from build123d import *

# Parameters (mm, degrees)
SKETCH_1_R          = 2.5
SKETCH_1_R_2        = 3
EXTRUDE_1_DEPTH     = 5
SKETCH_2_R          = 10
SKETCH_2_R_2        = 3
EXTRUDE_2_DEPTH     = 5
FILLET_1_R          = 0.3
CHAMFER_1_SIZE      = 0.5
CUT_EXTRUDE_1_REACH = 29.325
SKETCH_3_W          = 1
SKETCH_3_H          = 13.579366256
HOLE_WIZARD_M4_1_D  = 3.3


with BuildPart() as part:
    # 草图1 → 凸台-拉伸1 (new body)
    with BuildSketch(Plane(origin=(0, 0, 0), x_dir=(1, 0, 0), z_dir=(0, 1, 0))):
        with BuildLine():
            Line((-17.966197006, 5.136542547), (-7.985903938, 8.956859846))
            Line((-7.985903938, 8.956859846), (-7.985903938, 13.579366256))
            Line((-7.985903938, 13.579366256), (7.985903938, 13.579366256))
            Line((7.985903938, 13.579366256), (7.985903938, 8.956859846))
            Line((7.985903938, 8.956859846), (17.966197006, 5.136542547))
            ThreePointArc((17.966197006, 5.136542547), (21.495547327, -0.221268111), (17.546875, -5.277989933))
            Line((17.546875, -5.277989933), (1.435216594, -10))
            Line((1.435216594, -10), (-1.435216594, -10))
            Line((-1.435216594, -10), (-17.546875, -5.277989933))
            ThreePointArc((-17.546875, -5.277989933), (-21.495547327, -0.221268111), (-17.966197006, 5.136542547))
        make_face()
        with Locations(Location((-16, 0, 0), (0, 0, 270))):
            Circle(SKETCH_1_R, mode=Mode.SUBTRACT)
        with Locations(Location((0, 0, 0), (0, 0, 270))):
            Circle(SKETCH_1_R_2, mode=Mode.SUBTRACT)
        with Locations(Location((16, 0, 0), (0, 0, 90))):
            Circle(SKETCH_1_R, mode=Mode.SUBTRACT)
    extrude(amount=EXTRUDE_1_DEPTH)

    # 草图2 → 凸台-拉伸2 (add)
    with BuildSketch(Plane(origin=(0, 5, 0), x_dir=(1, 0, 0), z_dir=(0, 1, 0))):
        with Locations(Location((0, 0, 0), (0, 0, 270))):
            Circle(SKETCH_2_R)
        with Locations(Location((0, 0, 0), (0, 0, 270))):
            Circle(SKETCH_2_R_2, mode=Mode.SUBTRACT)
    extrude(amount=EXTRUDE_2_DEPTH)

    # 圆角1
    fillet_1_edges = [part.edges().sort_by_distance(p)[0] for p in [
        (0, 0, -13.579366256),
        (7.985903938, 0, -11.268113051),
        (-7.985903938, 2.5, -13.579366256),
        (7.985903938, 2.5, -13.579366256),
        (7.985903938, 5, -11.268113051),
        (0, 5, -13.579366256),
        (-7.985903938, 5, -11.268113051),
        (-7.985903938, 0, -11.268113051),
    ]]
    fillet(fillet_1_edges, radius=FILLET_1_R)

    # 倒角1
    chamfer_1_edges = [part.edges().sort_by_distance(p)[0] for p in [
        (0, 10, -10),
    ]]
    chamfer(chamfer_1_edges, length=CHAMFER_1_SIZE)

    # 草图3 → 切除-拉伸1 (cut, up to next)
    with BuildSketch(Plane(origin=(0, 10, 0), x_dir=(1, 0, 0), z_dir=(0, 1, 0)), mode=Mode.PRIVATE) as cut_extrude_1_sk1:
        with Locations((0, 6.789683128)):
            Rectangle(SKETCH_3_W, SKETCH_3_H)
    cut_extrude_1_tool1 = extrude(cut_extrude_1_sk1.sketch, amount=-CUT_EXTRUDE_1_REACH, mode=Mode.PRIVATE) & part.part
    add(cut_extrude_1_tool1.solids().sort_by_distance((0, 10, -6.789683))[0], mode=Mode.SUBTRACT)

    # M4 螺纹孔1 (through all)
    with Locations(Plane(origin=(-7.985903938, 2.5, -11.156859846), x_dir=(0, 0, -1), z_dir=(-1, 0, 0))):
        with Locations((0, 0)):
            Hole(HOLE_WIZARD_M4_1_D / 2)


solid = part.part
The listing builds one solid part. Answer for the finished solid, in the listing's coordinates (mm). A direction names the side the tool comes from. Give positions to 0.01 mm unless a question says otherwise; leave off trailing zeros. Write each loop counter-clockwise with the first axis right and the second up, starting at its lowest first coordinate (ties: lowest second). Pieces come first, ordered by that corner, then holes. Notation, with made-up numbers: (48, 10) - (57, 10) arc R20 ccw to (57, 25) - close; hole circle Ø3 at (31.25, 36.25). An arc over 180 degrees is marked (long way). Use a Markdown table: item, result.
1. For a pull along Y with two mould halves and no side action, classify faces 1 (the cylindrical face through (-18.44, 2.46, -0.54)), 2 (the cylindrical face through (4.295, 2.427, -12.805)), 3 (the flat face through (2.24, 10, -2.24)), 4 (the cylindrical face through (-4.191, 2.427, -12.805)) as released by +Y, released by -Y, zero draft, split by the parting line, or undercut.
Values follow:
| item | result |
|---|---|
| face 1 | zero draft |
| face 2 | undercut |
| face 3 | released by +Y |
| face 4 | undercut |
2. Find the intervals of material crossed by probe 1 along X at (y, z) = (2.8, 0); probe 2 along Y at (x, z) = (12.5, -4.5); probe 3 along Z at (x, y) = (-1.5, 1.5), in increasing order. Write a range as from..to.
Values follow:
| item | result |
|---|---|
| probe 1 | x = -21.5..-18.5, -13.5..-3, 3..13.5, 18.5..21.5 |
| probe 2 | y = 0..5 |
| probe 3 | z = -13.58..-12.47, -9.84..-2.6, 2.6..9.98 |
3. Section A-A on y = 2.5 is taken. Write down the section's boundary in (x, z), plus the area to 3 significant figures.
Values follow:
| item | result |
|---|---|
| outline | (-17.97, -5.14) - (-7.99, -8.96) - (-7.99, -9.51) - (-0.5, -9.51) - (-0.5, -2.96) arc R3 cw (long way) to (0.5, -2.96) - (0.5, -9.51) - (7.99, -9.51) - (7.99, -8.96) - (17.97, -5.14) arc R5.5 ccw to (17.55, 5.28) - (1.44, 10) - (-1.44, 10) - (-17.55, 5.28) arc R5.5 ccw to start; (-7.99, -13.28) arc R0.3 ccw to (-7.69, -13.58) - (-0.5, -13.58) - (-0.5, -12.81) - (-7.99, -12.81) - close; (0.5, -13.58) - (7.69, -13.58) arc R0.3 ccw to (7.99, -13.28) - (7.99, -12.81) - (0.5, -12.81) - close; hole circle Ø5 at (-16, 0); hole circle Ø5 at (16, 0) |
| area | 562 mm² |
4. Section D-D on x = -11 is taken. Write down the section's boundary in (y, z), plus the area to 3 significant figures.
Values follow:
| item | result |
|---|---|
| outline | (0, -7.8) - (5, -7.8) - (5, 7.2) - (0, 7.2) - close |
| area | 75.0 mm² |
5. Each of these flat-tipped pins is pushed along its axis until it touches: P1, Ø5, axis at x = 13, z = -8.5, coming from the +Y side; P2, Ø2, axis at x = 6.5, y = 8.5, coming from the -Z side; P3, Ø4, axis at y = 3, z = 7, coming from the -X side; P4, Ø2, axis at y = 2.5, z = -11.16, coming from the +X side. Where does it stop, or does it pass through?
Values follow:
| item | result |
|---|---|
| P1 | stops at y = 5 |
| P2 | stops at z = -8.35 |
| P3 | stops at x = -18.29 |
| P4 | passes through |
6. Section B-B on x = 16 is taken. Write down the section's boundary in (y, z), plus the area to 3 significant figures.
Values follow:
| item | result |
|---|---|
| outline | (0, -5.89) - (5, -5.89) - (5, -2.5) - (0, -2.5) - close; (0, 2.5) - (5, 2.5) - (5, 5.73) - (0, 5.73) - close |
| area | 33.1 mm² |
7. Section C-C on z = 1.5 is taken. Count the separate pieces of the cut face and the enclosed holes in it, plus the area to 3 significant figures.
Values follow:
| item | result |
|---|---|
| separate pieces | 4 |
| enclosed holes | 0 |
| area | 220 mm² |
8. A tool of negligible diameter and unlimited length cuts with its end or side. For faces 5 (the cylindrical face through (0, 7, 10)), 6 (the flat face through (-0.5, 5, -7)), 7 (the flat face through (7.986, 1, -13)), from which of +Z, -Z, +X, -X, +Y, -Y can it reach the whole face along a straight path? Write none if from no direction.
Values follow:
| item | result |
|---|---|
| face 5 | +Y |
| face 6 | -Z, +Y, -Y |
| face 7 | -Z, +X, +Y, -Y |
